Build history of the part. All positions in model axes, mm. Round coordinates to 2 decimals unless told otherwise and drop trailing zeros. Write each loop counter-clockwise with the first axis right and the second up, starting at its lowest first coordinate (ties: lowest second). Pieces come first, ordered by that corner, then holes.
1) Flat gauge pin, fed straight in: pin 1 (5.5 mm diameter, centred on x = -34.5, z = -34.5, fed in from -Y). Where does the tip first touch, or does it go through?
2) Pull direction Z, two halves, no side cores. Call faces 1 (the cylindrical face through (31.5, 2.5, 34.4)), 2 (the cylindrical face through (31.5, 2.5, -34.6)), 3 (the flat face through (-1, 5, -1)), 4 (the cylindrical face through (-41.64, 2.54, -41.6)): +Z half, -Z half, draft (parallel to the pull), parting line (faces both ways), or undercut.
3) Saw through at B-B (x = -34.5). Write the cut outline in (y, z).
4) Saw through at A-A (z = -34.5). Write the cut outline in (x, y), plus the area to 3 significant figures.
5) Saw through at C-C (y = 1.3). Write the cut outline in (x, z), plus the area to 3 significant figures.
6) Wall check: probe 1 along X at (y, z) = (3.3, 34.5); probe 2 along Z at (x, y) = (-36.5, 4.55). Give the ranges that are in metal, low to high.
from build123d import *

# Parameters (mm, degrees)
SKETCH1_W           = 85
SKETCH1_H           = 85
BOSS_EXTRUDE1_DEPTH = 5
FILLET1_R           = 3
SKETCH2_R           = 3
CUT_EXTRUDE1_DEPTH  = 6


with BuildPart() as part:
    # Sketch1 → Boss-Extrude1 (new body)
    with BuildSketch(Plane(origin=(0, 0, 0), x_dir=(1, 0, 0), z_dir=(0, 1, 0))):
        Rectangle(SKETCH1_W, SKETCH1_H)
    extrude(amount=BOSS_EXTRUDE1_DEPTH)

    # Fillet1
    fillet1_edges = [part.edges().sort_by_distance(p)[0] for p in [
        (42.5, 2.5, 42.5),
        (-42.5, 2.5, 42.5),
        (-42.5, 2.5, -42.5),
        (42.5, 2.5, -42.5),
    ]]
    fillet(fillet1_edges, radius=FILLET1_R)

    # Sketch2 → Cut-Extrude1 (cut, through all)
    with BuildSketch(Plane(origin=(0, 5, 0), x_dir=(1, 0, 0), z_dir=(0, 1, 0))):
        with Locations((-34.5, 34.5)):
            Circle(SKETCH2_R)
        with Locations((-34.5, -34.5)):
            Circle(SKETCH2_R)
        with Locations((34.5, -34.5)):
            Circle(SKETCH2_R)
        with Locations((34.5, 34.5)):
            Circle(SKETCH2_R)
    extrude(amount=-CUT_EXTRUDE1_DEPTH, mode=Mode.SUBTRACT)


solid = part.part
Evaluation:
1. pin 1: passes through
2. face 1: undercut
2. face 2: undercut
2. face 3: draft
2. face 4: -Z half
3. outline: (0, -42.5) - (5, -42.5) - (5, -37.5) - (0, -37.5) - close; (0, -31.5) - (5, -31.5) - (5, 31.5) - (0, 31.5) - close; (0, 37.5) - (5, 37.5) - (5, 42.5) - (0, 42.5) - close
4. outline: (-42.5, 0) - (-37.5, 0) - (-37.5, 5) - (-42.5, 5) - close; (-31.5, 0) - (31.5, 0) - (31.5, 5) - (-31.5, 5) - close; (37.5, 0) - (42.5, 0) - (42.5, 5) - (37.5, 5) - close
4. area: 365 mm2
5. outline: (-42.5, -39.5) arc R3 ccw to (-39.5, -42.5) - (39.5, -42.5) arc R3 ccw to (42.5, -39.5) - (42.5, 39.5) arc R3 ccw to (39.5, 42.5) - (-39.5, 42.5) arc R3 ccw to (-42.5, 39.5) - close; hole circle Ø6 at (-34.5, -34.5); hole circle Ø6 at (-34.5, 34.5); hole circle Ø6 at (34.5, -34.5); hole circle Ø6 at (34.5, 34.5)
5. area: 7,100 mm2
6. probe 1: x = -42.5 to -37.5, -31.5 to 31.5, 37.5 to 42.5
6. probe 2: z = -42.5 to -36.74, -32.26 to 32.26, 36.74 to 42.5
